Autodesk Inventor part; units mm, degrees
ref_plane "YZ Plane" through (0, 0, 0) normal (1, 0, 0) x (0, 1, 0)
ref_plane "XZ Plane" through (0, 0, 0) normal (0, 1, 0) x (-1, 0, 0)
ref_plane "XY Plane" through (0, 0, 0) normal (0, 0, 1) x (1, 0, 0)
sketch "Sketch1" plane through (0, 0, 0) normal (0, 0, 1) x (1, 0, 0)
  line L0 (0, 0) -> (-50, 0)
  line L1 (0, 0) -> (0, 50)
  arc A0 (0, 50) -> (-50, 0) centre (0, 0) ccw
  dimension "d0" = 50
extrude "Wafer" add sketch "Sketch1" along normal blind 0.525
fillet "OutsideEdge" radius 0.1 1 edges at (-35.3553, 35.3553, 0.525)
sketch "Sketch3" plane through (0, 0, 0) normal (0, 0, -1) x (-1, 0, 0)
  line L0 (0, 50) -> (0, 0)
  arc A0 (49.9, 0) -> (0, 49.9) centre (0, 0) ccw
  line L1 (0, 0) -> (49.9, 0)
  line L2 (0, 49.9) -> (0, 0)
extrude "Wax" add sketch "Sketch3" along normal blind 0.25
sketch "Sketch4" plane through (0, 0, 0.525) normal (0, 0, 1) x (1, 0, 0)
  line L0 (0, 0) -> (-49.9, 0)
  line L1 (0, 49.9) -> (0, 0)
  line L2 (-24.5, 24.5) -> (-15.5, 24.5) construction
  line L3 (-15.5, 24.5) -> (-15.5, 15.5) construction
  line L4 (-15.5, 15.5) -> (-24.5, 15.5) construction
  line L5 (-24.5, 15.5) -> (-24.5, 24.5) construction
  line L6 (-24.5, 20) -> (-15.5, 20) construction
  line L7 (-20, 24.5) -> (-20, 15.5) construction
  line L8 (-25, 25) -> (-15, 25)
  line L9 (-15, 25) -> (-15, 15)
  line L10 (-15, 15) -> (-25, 15)
  line L11 (-25, 15) -> (-25, 25)
  line L12 (-20, 25) -> (-20, 24.5) construction
  line L13 (-15, 20) -> (-15.5, 20) construction
  line L14 (-27.75, 27.75) -> (-27.25, 27.75) construction
  line L15 (-27.25, 27.75) -> (-27.25, 27.25) construction
  line L16 (-27.25, 27.25) -> (-27.75, 27.25) construction
  line L17 (-27.75, 27.25) -> (-27.75, 27.75) construction
  line L18 (-27.75, 27.5) -> (-27.25, 27.5) construction
  line L19 (-27.5, 27.75) -> (-27.5, 27.25) construction
  line L20 (-27.75, 27.75) -> (-27.75, 28.25)
  line L21 (-27.75, 28.25) -> (-27.25, 28.25)
  line L22 (-27.25, 28.25) -> (-27.25, 27.75)
  line L23 (-27.25, 27.75) -> (-26.75, 27.75)
  line L24 (-26.75, 27.75) -> (-26.75, 27.25)
  line L25 (-26.75, 27.25) -> (-27.25, 27.25)
  line L26 (-27.25, 27.25) -> (-27.25, 26.75)
  line L27 (-27.25, 26.75) -> (-27.75, 26.75)
  line L28 (-27.75, 26.75) -> (-27.75, 27.25)
  line L29 (-27.75, 27.25) -> (-28.25, 27.25)
  line L30 (-28.25, 27.25) -> (-28.25, 27.75)
  line L31 (-28.25, 27.75) -> (-27.75, 27.75)
  point P0 (-20, 20)
  point P1 (-20, 20)
  point P2 (-20, 20)
  dimension "d8" = 20
  dimension "d9" = 20
  dimension "d10" = 9
  dimension "d11" = 10
  dimension "d14" = 0.5
  dimension "d15" = 2.5
  dimension "d16" = 2.5
extrude "Cutout" cut sketch "Sketch4" against normal blind 0.1 draft -57.6
properties part number "carrier-wafer"
Source: CAD feature listing. Evaluate the final solid. Frame: model axes, mm. Round coordinates to 2 decimals unless told otherwise and drop trailing zeros. Loops run counter-clockwise (first coordinate to the right, second up) from the corner with the lowest first, then second, coordinate; pieces in that order, holes last. Notation, with made-up numbers: M -37,50 L 8,50 A28 ccw 8,81 Z; hole C 49.25,-39 d4. An arc over 180 degrees is marked long. Return JSON: item names as keys, results as strings. Group by question number.
1. Material intervals for line 1 along Z through (x, y) = (-18, 19.5) (3 decimals); line 2 along X through (y, z) = (31, 0.05); line 3 along Y through (x, z) = (-21, -0.1), sorted ascending. Write a range as from..to.
2. Section query A-A on z = 0.3. Output: boundary loops of the cut face in (x, y).
3. Mould query, pull axis Y, two halves, no side actions, for faces 1 (the face through (-20, 20, 0.425)), 2 (the face through (-19, 20, -0.25)), 3 (the face through (-35.742, 34.964, 0.21)). Classes: released by +Y, released by -Y, zero draft, split by the parting line, or undercut.
4. Pin query (flat end, axial travel): pin 1 (5 mm diameter, centred on x = -18, y = 19, fed in from +Z) (3 decimals). Return the tip coordinate at first contact, or that it passes through.
Checks:
{
 "1": {"line 1": "z = -0.25..0.425", "line 2": "x = -39.23..0", "line 3": "y = 0..45.27"},
 "2": {"outline": "M -50,0 L 0,0 L 0,50 A50 ccw Z"},
 "3": {"face 1": "undercut", "face 2": "zero draft", "face 3": "released by +Y"},
 "4": {"pin 1": "stops at z = 0.425"}
}
